from build123d import *

# Parameters (mm, degrees)
SKETCH3_W           = 20
SKETCH3_H           = 70
BOSS_EXTRUDE3_DEPTH = 5
CUT_EXTRUDE2_DEPTH  = 2
SKETCH6_R           = 3.57
CUT_EXTRUDE3_DEPTH  = 3
SKETCH7_R           = 1.05
SKETCH7_W           = 12.3
SKETCH7_H           = 22.7
CUT_EXTRUDE4_DEPTH  = 5


with BuildPart() as part:
    # Sketch3 → Boss-Extrude3 (new body)
    with BuildSketch(Plane.XY):
        Rectangle(SKETCH3_W, SKETCH3_H)
    extrude(amount=BOSS_EXTRUDE3_DEPTH)

    # Sketch4 → Cut-Extrude2 (cut)
    with BuildSketch(Plane.XY.offset(5)):
        with BuildLine():
            Line((-2.85, 24.850023256), (-1.8, 12.795667197))
            Line((-1.8, 12.795667197), (1.8, 12.795667197))
            Line((1.8, 12.795667197), (2.85, 24.850023256))
            ThreePointArc((2.85, 24.850023256), (0, 23.43), (-2.85, 24.850023256))
        make_face()
        with BuildLine():
            Line((1.8, 12.795667197), (-1.8, 12.795667197))
            ThreePointArc((-1.8, 12.795667197), (0, 10.995667197), (1.8, 12.795667197))
        make_face()
        with BuildLine():
            ThreePointArc((3.57, 27), (-1.133666618, 30.385217866), (-2.85, 24.850023256))
            Line((-2.85, 24.850023256), (2.85, 24.850023256))
            ThreePointArc((2.85, 24.850023256), (3.385217866, 25.866333382), (3.57, 27))
        make_face()
        with BuildLine():
            Line((2.85, 24.850023256), (-2.85, 24.850023256))
            ThreePointArc((-2.85, 24.850023256), (0, 23.43), (2.85, 24.850023256))
        make_face()
    extrude(amount=-CUT_EXTRUDE2_DEPTH, mode=Mode.SUBTRACT)

    # Sketch6 → Cut-Extrude3 (cut)
    with BuildSketch(Plane.XY.offset(3)):
        with Locations((0, 27)):
            Circle(SKETCH6_R)
    extrude(amount=-CUT_EXTRUDE3_DEPTH, mode=Mode.SUBTRACT)

    # Sketch7 → Cut-Extrude4 (cut)
    with BuildSketch(Plane.XY.offset(5)):
        with Locations((0, -5.33)):
            Circle(SKETCH7_R)
        with Locations((0, -32.67)):
            Circle(SKETCH7_R)
        with Locations((0, -19)):
            Rectangle(SKETCH7_W, SKETCH7_H)
    extrude(amount=-CUT_EXTRUDE4_DEPTH, mode=Mode.SUBTRACT)


solid = part.part
Could you check a few things on this model? Use its own coordinates, in mm. A direction names the side the tool comes from. Round coordinates to 2 decimals unless told otherwise and drop trailing zeros. Write each loop counter-clockwise with the first axis right and the second up, starting at its lowest first coordinate (ties: lowest second). Pieces come first, ordered by that corner, then holes. Notation, with made-up numbers: (69.5, -34.75) - (125.5, -34.75) arc R18 cw to (125.5, -6.75) - close; hole circle Ø7 at (19, 31). An arc over 180 degrees is marked (long way). Use a Markdown table: item, result.
Q1. I want a section at A-A (x = 0). List the corners of the cut face in (y, z) for me, plus the area to 3 significant figures.
Output values:
| item | result |
|---|---|
| outline | (-35, 0) - (-33.72, 0) - (-33.72, 5) - (-35, 5) - close; (-31.62, 0) - (-30.35, 0) - (-30.35, 5) - (-31.62, 5) - close; (-7.65, 0) - (-6.38, 0) - (-6.38, 5) - (-7.65, 5) - close; (-4.28, 0) - (23.43, 0) - (23.43, 3) - (11, 3) - (11, 5) - (-4.28, 5) - close; (30.57, 0) - (35, 0) - (35, 5) - (30.57, 5) - close |
| area | 155 mm2 |
Q2. I want a section at C-C (z = 3.85). List the corners of the cut face in (x, y) for me, plus the area to 3 significant figures.
Output values:
| item | result |
|---|---|
| outline | (-10, -35) - (10, -35) - (10, 35) - (-10, 35) - close; hole (-6.15, -30.35) - (6.15, -30.35) - (6.15, -7.65) - (-6.15, -7.65) - close; hole (-2.85, 24.85) - (-1.8, 12.8) arc R1.8 ccw to (1.8, 12.8) - (2.85, 24.85) arc R3.57 ccw (long way) to start; hole circle Ø2.1 at (0, -32.67); hole circle Ø2.1 at (0, -5.33) |
| area | 1,020 mm2 |
Q3. For pin 1 (1.7 mm diameter, centred on x = 0, y = -32.67, fed in from -Z); pin 2 (3 mm diameter, centred on x = 0.5, y = 20.5, fed in from +Z), each with a flat end and sliding along its axis, tell me the tip position at first contact or that it passes through.
Output values:
| item | result |
|---|---|
| pin 1 | through |
| pin 2 | z = 3 |
Q4. I want a section at D-D (z = 1). List the corners of the cut face in (x, y) for me.
Output values:
| item | result |
|---|---|
| outline | (-10, -35) - (10, -35) - (10, 35) - (-10, 35) - close; hole (-6.15, -30.35) - (6.15, -30.35) - (6.15, -7.65) - (-6.15, -7.65) - close; hole circle Ø7.14 at (0, 27); hole circle Ø2.1 at (0, -32.67); hole circle Ø2.1 at (0, -5.33) |
Q5. For faces 4 (the flat face through (-6.15, -19, 3)), 5 (the flat face through (0, 0, 0)), 6 (the flat face through (-2.332, 18.907, 4.014)), which set-ups out of +Z, -Z, +X, -X, +Y, -Y let a thin tool reach every point of the face, with its end or its side?
Output values:
| item | result |
|---|---|
| face 4 | +Z, -Z |
| face 5 | -Z, +X, -X, +Y, -Y |
| face 6 | +Z |
Q6. Please list where these lines run through material, in increasing order: L1, parallel to Y at x = 0, z = 3.9; L2, parallel to Y at x = 0, z = 1.95; L3, parallel to X at y = 27, z = 0.8.
Output values:
| item | result |
|---|---|
| L1 | -35 to -33.72, -31.62 to -30.35, -7.65 to -6.38, -4.28 to 11, 30.57 to 35 |
| L2 | -35 to -33.72, -31.62 to -30.35, -7.65 to -6.38, -4.28 to 23.43, 30.57 to 35 |
| L3 | -10 to -3.57, 3.57 to 10 |
Q7. Thinking about a two-plate mould opening in X: for faces 1 (the flat face through (0, -35, 2)), 2 (the flat face through (-10, 0, 2)), 3 (the flat face through (6.15, -19, 3)), which applies, released by +X, released by -X, zero draft, split by the parting line, or undercut?
Output values:
| item | result |
|---|---|
| face 1 | zero draft |
| face 2 | released by -X |
| face 3 | undercut |
Q8. I want a section at B-B (y = -16). List the corners of the cut face in (x, z) for me, plus the area to 3 significant figures.
Output values:
| item | result |
|---|---|
| outline | (-10, 0) - (-6.15, 0) - (-6.15, 5) - (-10, 5) - close; (6.15, 0) - (10, 0) - (10, 5) - (6.15, 5) - close |
| area | 38.5 mm2 |
